Model file for the job. Use its own axes, mm. A direction names the side the tool comes from. Coordinates: 2 decimals unless noted, no trailing zeros. Order: outer loops, then holes, each group sorted by start corner. A loop starts at its lowest first (then second) coordinate and runs counter-clockwise, first axis right, second up.
Autodesk Inventor part; units mm, degrees
ref_plane "YZ Plane" through (0, 0, 0) normal (1, 0, 0) x (0, 1, 0)
ref_plane "XZ Plane" through (0, 0, 0) normal (0, 1, 0) x (-1, 0, 0)
ref_plane "XY Plane" through (0, 0, 0) normal (0, 0, 1) x (1, 0, 0)
sketch "Náčrt1" plane through (0, 0, 0) normal (0, 0, 1) x (1, 0, 0)
  line L0 (-200, -200) -> (200, -200)
  line L1 (200, -200) -> (200, 200)
  line L2 (200, 200) -> (-200, 200)
  line L3 (-200, 200) -> (-200, -200)
  line L4 (-200, -200) -> (200, 200) construction
  line L5 (200, -200) -> (-200, 200) construction
  circle A0 centre (0, 0) radius 400
  dimension "d6" = 800
  dimension "d7" = 400
extrude "Vysunutí1" add sketch "Náčrt1" along normal blind 600
sketch "Náčrt2" plane through (0, 0, 0) normal (0, 0, -1) x (-1, 0, 0)
  line L0 (200, 200) -> (200, -200)
  line L1 (200, -200) -> (-200, -200)
  line L2 (-200, -200) -> (-200, 200)
  line L3 (-200, 200) -> (200, 200)
  circle A0 centre (0, 0) radius 400
  circle A1 centre (0, 0) radius 450
  dimension "d8" = 900
extrude "Vysunutí2" add sketch "Náčrt2" along normal blind 50 contours A0 | A1
sketch "Náčrt3" plane through (0, 0, 600) normal (0, 0, 1) x (1, 0, 0)
  line L0 (251.7841, 450) -> (-248.2159, 450)
  line L1 (-248.2159, 450) -> (-248.2159, 350)
  line L2 (-248.2159, 350) -> (251.7841, 350)
  line L3 (251.7841, 350) -> (251.7841, 450)
  circle A0 centre (0, 0) radius 400
  dimension "d11" = 350
  dimension "d12" = 100
  dimension "d13" = 500
extrude "Vysunutí3" cut sketch "Náčrt3" against normal blind 50 contours L3 L2 A0 L1 L0 | L2 A0 picked at (-56.548, 354.0814)
sketch "Náčrt4" plane through (0, 0, -50) normal (0, 0, -1) x (-1, 0, 0)
  line L0 (200, -200) -> (-200, -200)
  line L1 (200, 200) -> (200, -200)
  line L2 (-200, 200) -> (200, 200)
  line L3 (-200, -200) -> (-200, 200)
  line L4 (-250, -250) -> (250, -250)
  line L5 (250, -250) -> (250, 250)
  line L6 (250, 250) -> (-250, 250)
  line L7 (-250, 250) -> (-250, -250)
  point P0 (0, 0)
  dimension "d16" = 50
extrude "Vysunutí4" add sketch "Náčrt4" along normal blind 600
properties part number "B3-C"
Q1. Mould opens along Y. For faces 4 (the face through (-3, -200, -16)), 5 (the face through (449.565, -19.786, -24.65)), 6 (the face through (3, -250, -346)) say: pulls with the +Y half, pulls with the -Y half, needs draft (parallel to the pull), parting line crosses it, or undercut.
Established:
face 4: undercut
face 5: parting line crosses it
face 6: pulls with the -Y half
Q2. Which spindle directions (+Z, -Z, +X, -X, +Y, -Y) get a long thin tool onto all of the face, cutting with end or side? Do faces 1 (the face through (-250, -3, -346)), 2 (the face through (250, 3, -346)), 3 (the face through (-3, 350, 575)). Say none if no direction does.
Established:
face 1: -Z, -X, +Y, -Y
face 2: -Z, +X, +Y, -Y
face 3: +Z, +X, -X, +Y
Q3. Cut at C-C, the plane x = 0. List the corners of the cut face in (y, z), plus the area to 4 significant figures.
Established:
outline: (-450, -50) - (-250, -50) - (-250, -650) - (-200, -650) - (-200, 600) - (-400, 600) - (-400, 0) - (-450, 0) - close; (200, -650) - (250, -650) - (250, -50) - (450, -50) - (450, 0) - (400, 0) - (400, 550) - (350, 550) - (350, 600) - (200, 600) - close
area: 322,500 mm2
Q4. Probe line 1 (Y direction, x = 102, z = -502.5); line 2 (X direction, y = 3.5, z = 340). List the from-to ranges inside material, lowest first.
Established:
line 1: y = -250 to -200, 200 to 250
line 2: x = -399.98 to -200, 200 to 399.98
Q5. Cut at B-B, the plane z = 134.5. List the corners of the cut face in (x, y).
Established:
outline: circle Ø800 at (0, 0); hole (-200, -200) - (200, -200) - (200, 200) - (-200, 200) - close
Q6. Drop flat-ended pins along their axis: P1, Ø2, axis at y = 167.5, z = -40, coming from the +X side; P2, Ø2, axis at x = -353, y = -57.5, coming from the -Z side; P3, Ø5, axis at y = -200.5, z = 343, coming from the +X side. Give the stop position or say it passes through.
Established:
P1: stops at x = 418.06
P2: stops at z = -50
P3: stops at x = 347.56
Q7. Cut at D-D, the plane y = -95.5. List the corners of the cut face in (x, z).
Established:
outline: (-439.75, -50) - (-250, -50) - (-250, -650) - (-200, -650) - (-200, 600) - (-388.43, 600) - (-388.43, 0) - (-439.75, 0) - close; (200, -650) - (250, -650) - (250, -50) - (439.75, -50) - (439.75, 0) - (388.43, 0) - (388.43, 600) - (200, 600) - close
Q8. Cut at A-A, the plane y = 0. List the corners of the cut face in (x, z).
Established:
outline: (-450, -50) - (-250, -50) - (-250, -650) - (-200, -650) - (-200, 600) - (-400, 600) - (-400, 0) - (-450, 0) - close; (200, -650) - (250, -650) - (250, -50) - (450, -50) - (450, 0) - (400, 0) - (400, 600) - (200, 600) - close
